Verification items for this drawing (mm, ordinates from the low corner). A direction names the side the tool comes from. Round coordinates to 2 decimals unless told otherwise and drop trailing zeros. Loops run counter-clockwise (first coordinate to the right, second up) from the corner with the lowest first, then second, coordinate; pieces in that order, holes last. Notation, with made-up numbers: M -40,64.5 L 11,64.5 A22 ccw 11,87.5 Z; hole C 66,3.25 d2. An arc over 180 degrees is marked long. Write item = value, one per line. Start each with the question number.
(1) Cross-section at A-A on y = 6. Record the boundary of the cut face in (x, z).
(2) Cross-section at B-B on x = 12.25. Record the boundary of the cut face in (y, z).
(3) Set-up check for the marked faces 1, 2, 3, 4 and 5: record each of +Z, -Z, +X, -X, +Y, -Y from which the full face is reachable in a straight line by a thin tool's end or side.
(4) Scan lines: L1, parallel to Y at x = 2.5, z = 9; L2, parallel to Z at x = 10.75, y = 8.75; L3, parallel to X at y = 9.5, z = 5.5. Record each from-to range of solid material in increasing order. Write a range as from..to.
(5) Go/stop test with flat-tipped pins: P1, Ø2.5, axis at y = 7, z = 5.5, coming from the -X side; P2, Ø3, axis at y = 4, z = 1, coming from the -X side; P3, Ø6.5, axis at x = 7, y = 8, coming from the -Z side; P4, Ø4, axis at x = 7, y = 9.5, coming from the +Z side. Record where each tip stops, or that it passes through.
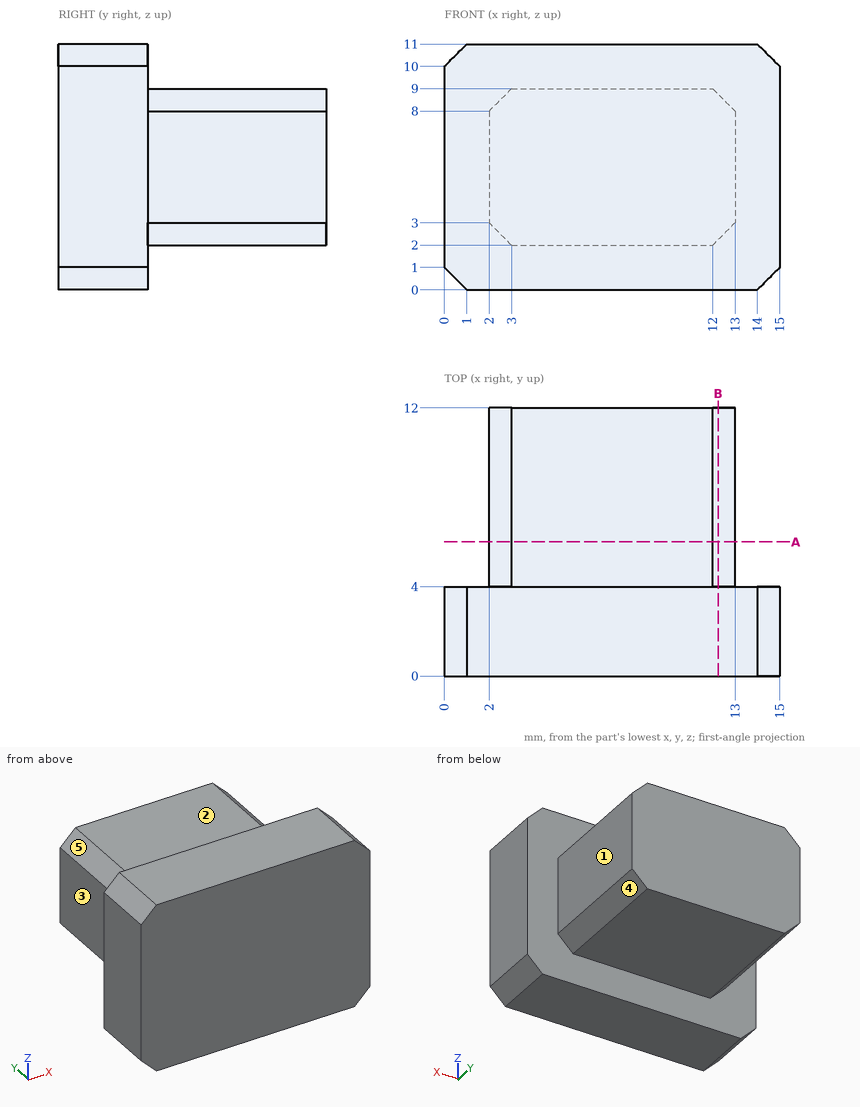
Result:
q1.outline = M 2,3 L 3,2 L 12,2 L 13,3 L 13,8 L 12,9 L 3,9 L 2,8 Z
q2.outline = M 0,0 L 4,0 L 4,2.25 L 12,2.25 L 12,8.75 L 4,8.75 L 4,11 L 0,11 Z
q3.face_1 = +Z, -Z, +X, +Y
q3.face_2 = +Z, +X, -X, +Y
q3.face_3 = +Z, -Z, -X, +Y
q3.face_4 = -Z, +X, +Y
q3.face_5 = +Z, -X, +Y
q4.L1 = 0..4
q4.L2 = 2..9
q4.L3 = 2..13
q5.P1 = 2
q5.P2 = 0
q5.P3 = 2
q5.P4 = 9
